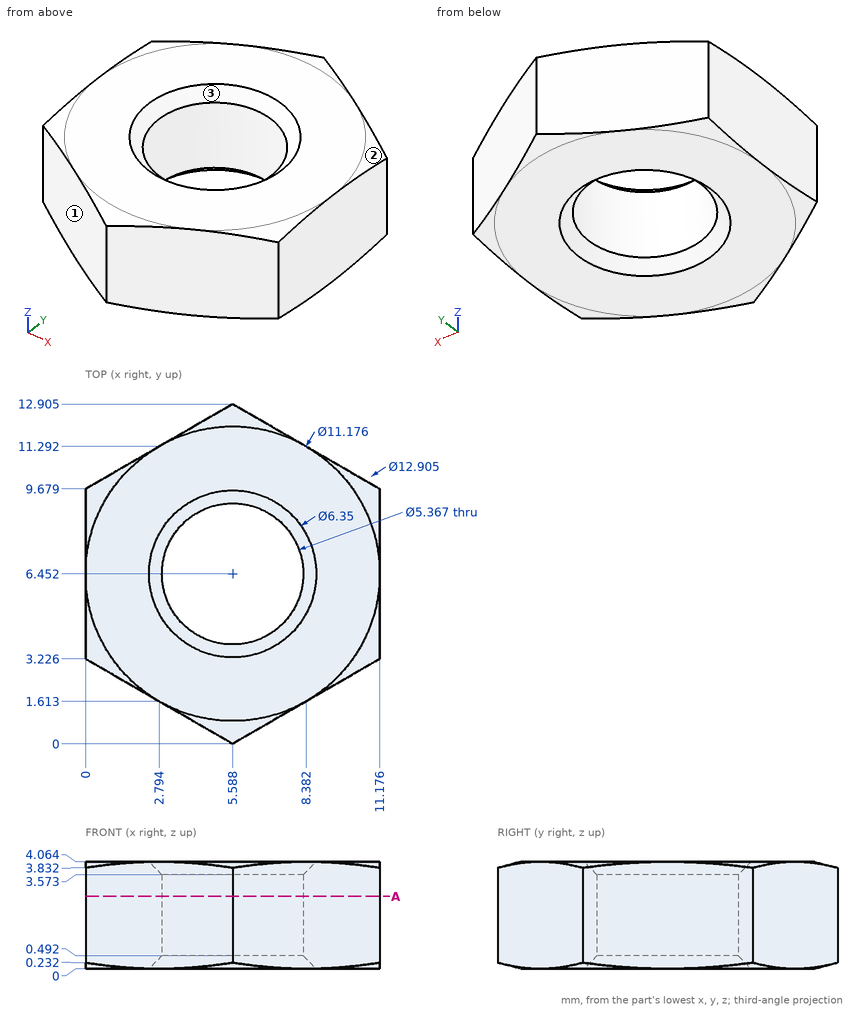
Print and shaded views of the part. All mm, measured from the part's lowest x, y and z. Give positions to 0.01 mm unless a question says otherwise; leave off trailing zeros. Loops run counter-clockwise (first coordinate to the right, second up) from the corner with the lowest first, then second, coordinate; pieces in that order, holes last. Notation, with made-up numbers: (88.25, 75) -> (137.25, 75) arc R25 cw to (137.25, 113) -> close; hole circle Ø1 at (22, 85). An arc over 180 degrees is marked (long way). Use CSV: the item, a comma, the result in double quotes. Start each with the question number.
1) Mould opens along X. For the marked faces 1, 2 and 3 say: released by +X, released by -X, zero draft, split by the parting line, or undercut.
2) Slice it at A-A on z = 2.75. Give the cut face in (x, y) (1 decimal).
3) Wall check: line 1 (Y direction, x = 4.5, z = 0.55) (1 decimal); line 2 (Y direction, x = 8, z = 0.9) (1 decimal); line 3 (X direction, y = 7.5, z = 2.2) (1 decimal). Give the ranges that are in metal, low to high.
4) Flat gauge pin, fed straight in: pin 1 Ø1 at (x, z) = (2, 0.5) entering from -Y. Where does the tip first touch, or does it go through?
Computed values:
1,face 1,"released by -X"
1,face 2,"released by +X"
1,face 3,"undercut"
2,outline,"(0, 3.2) -> (5.6, 0) -> (11.2, 3.2) -> (11.2, 9.7) -> (5.6, 12.9) -> (0, 9.7) -> close; hole circle Ø5.4 at (5.6, 6.5)"
3,line 1,"y = 0.6 to 4, 8.9 to 12.3"
3,line 2,"y = 1.4 to 5.3, 7.6 to 11.5"
3,line 3,"x = 0 to 3.1, 8.1 to 11.2"
4,pin 1,"stops at y = 1.78"
